For this review, take the finished solid that the model builds, in its own axes (mm). A direction names the side the tool comes from. Coordinates: 2 decimals unless noted, no trailing zeros. Order: outer loops, then holes, each group sorted by start corner. A loop starts at its lowest first (then second) coordinate and runs counter-clockwise, first axis right, second up. Notation, with made-up numbers: M -31,23 L 9,23 A13 cw 9,38 Z; hole C 89,76.25 d4. An arc over 180 degrees is marked long. Use CSV: the item, a comma, the result in double quotes.
Autodesk Inventor part; units mm, degrees
ref_plane "YZ Plane" through (0, 0, 0) normal (1, 0, 0) x (0, 1, 0)
ref_plane "XZ Plane" through (0, 0, 0) normal (0, 1, 0) x (-1, 0, 0)
ref_plane "XY Plane" through (0, 0, 0) normal (0, 0, 1) x (1, 0, 0)
ref_plane "Plano de trabajo1" through (0, 0, 0) normal (0, 0, 1) x (1, 0, 0)
sketch "Boceto1" plane through (0, 0, 0) normal (0, 0, 1) x (1, 0, 0)
  line L0 (0, 0) -> (0, -3) construction
  line L1 (20, -3) -> (0, -3) construction
  line L2 (20, 0) -> (20, -3) construction
  line L3 (20, 0) -> (-49, 0)
  line L4 (-49, 0) -> (-49, 85) construction
  line L5 (-49, 85) -> (20, 85) construction
  line L6 (20, 85) -> (20, 0) construction
  line L7 (0, 0) -> (0, -1)
  line L8 (20, -1) -> (20, 0)
  line L9 (18, -3) -> (2, -3)
  arc A0 (0, -1) -> (2, -3) centre (2, -1) ccw
  arc A1 (18, -3) -> (20, -1) centre (18, -1) ccw
  line L10 (20, 0) -> (35.1716, 0)
  line L11 (40, 0) -> (40, 20) construction
  line L12 (40, 20) -> (20, 20) construction
  line L13 (20, 20) -> (20, 0)
  line L14 (-34, 0) -> (-34, -3) construction
  circle A2 centre (-39, 10.2728) radius 1.55
  line L15 (40, 0) -> (20, 20)
  line L16 (20, 20) -> (-49, 20)
  line L17 (-20, 20) -> (-39, 85)
  line L18 (-49, 0) -> (-49, 85)
  line L19 (-39, 85) -> (-49, 85)
  line L20 (40, 0) -> (20, 0)
  circle A3 centre (-42.7477, 80) radius 1.4 construction
  circle A4 centre (-42.7477, 80) radius 1.55
  point P0 (35.1716, 0)
  dimension "d0" = 2
  dimension "d1" = 20
  dimension "d2" = 20
  dimension "d4" = 85
  dimension "d5" = 15
  dimension "d6" = 3.1
  dimension "d8" = 45
  dimension "d9" = 0
  dimension "d12" = 40
  dimension "d13" = 10
  dimension "d28" = 3.1
extrude "Extrusión1" add sketch "Boceto1" along normal blind 3.1
fillet "Empalme1" radius 2 1 edges at (40, 0, 1.55)
fillet "Empalme2" radius 12 1 edges at (-49, 0, 1.55)
fillet "Empalme3" radius 4 1 edges at (20, 20, 1.55)
fillet "Empalme4" radius 12 1 edges at (-20, 20, 1.55)
fillet "Empalme5" radius 5 2 edges at (-39, 85, 1.55) (-49, 85, 1.55)
sketch "Boceto2" plane through (0, 0, 3.1) normal (0, 0, 1) x (1, 0, 0)
  circle A0 centre (15, 15) radius 1.6 construction
  circle A1 centre (5, 15) radius 1.6 construction
  arc A2 (-44, 85) -> (-49, 80) centre (-44, 80) ccw construction
  arc A3 (-37.9485, 81.4028) -> (-42.7477, 85) centre (-42.7477, 80) ccw construction
  point P0 (0, 0)
hole "Agujero1" at (5, 15, 3.1) at (15, 15, 3.1) direction (0, 0, -1) diameter 3 end through all
equation "\"d14\" = d28"
properties part number "ParedLateralGrua1"
Item 1: Clearance check with flat-ended pins moving along their axes: pin 1 Ø1.6 at (x, z) = (-20, 2) entering from -Y; pin 2 Ø0.5 at (y, z) = (-0.5, 2.5) entering from -X; pin 3 Ø0.8 at (y, z) = (-0.5, 1) entering from +X. State where each tip first meets the part, or that it passes through.
Solutions:
pin 1,"y = 0"
pin 2,"x = 0"
pin 3,"x = 20"
Item 2: For faces 1 (the face through (-18, 0, 2)), 2 (the face through (27, 0, 2)), 3 (the face through (19.89, 19.69, 1.57)), list the 3-axis set-ups (+Z, -Z, +X, -X, +Y, -Y) from which the entire face can be reached by the end or side of a thin tool; tool diameter is ignored.
Solutions:
face 1,"+Z, -Z, -X, -Y"
face 2,"+Z, -Z, +X, -Y"
face 3,"+Z, -Z, +X, +Y"
Item 3: To check wall thickness, follow line 1 along X through (y, z) = (15, 2.2); line 2 along Y through (x, z) = (-9, 0.3); line 3 along Y through (x, z) = (28, 1.9). State the ranges of each line that lie inside material, in increasing order. Write a range as [from, to].
Solutions:
line 1,"[-49, 3.5], [6.5, 13.5], [16.5, 25]"
line 2,"[0, 20]"
line 3,"[0, 12]"
Item 4: Add section D-D on x = 27. State the section outline as (y, z) points, and give its area (3 significant figures).
Solutions:
outline,"M 0,0 L 13,0 L 13,3.1 L 0,3.1 Z"
area,"40.3 mm^2"
Item 5: Add section A-A on y = 15. State the section outline as (x, z) points.
Solutions:
outline,"M -49,0 L 3.5,0 L 3.5,3.1 L -49,3.1 Z; M 6.5,0 L 13.5,0 L 13.5,3.1 L 6.5,3.1 Z; M 16.5,0 L 25,0 L 25,3.1 L 16.5,3.1 Z"
Item 6: Add section C-C on z = 0.6. State the section outline as (x, y) points, and give its area (3 significant figures).
Solutions:
outline,"M -49,12 A12 ccw -37,0 L 0,0 L 0,-1 A2 ccw 2,-3 L 18,-3 A2 ccw 20,-1 L 20,0 L 35.17,0 A2 ccw 36.59,3.41 L 21.17,18.83 A4 ccw 18.34,20 L -11.01,20 A12 cw -22.52,28.63 L -37.95,81.4 A5 ccw -42.75,85 L -44,85 A5 ccw -49,80 Z; hole C -42.75,80 d3.1; hole C -39,10.27 d3.1; hole C 5,15 d3; hole C 15,15 d3"
area,"2,850 mm^2"
Item 7: Draft analysis for pull direction Y (two halves, no side actions). For faces 4 (the face through (10, -3, 2)), 5 (the face through (4.93, 16.5, 1.53)), 6 (the face through (-49, 46, 2)), state which applies: released by +Y, released by -Y, zero draft, split by the parting line, or undercut.
Solutions:
face 4,"released by -Y"
face 5,"undercut"
face 6,"zero draft"
Item 8: Add section B-B on x = 5. State the section outline as (y, z) points.
Solutions:
outline,"M -3,0 L 13.5,0 L 13.5,3.1 L -3,3.1 Z; M 16.5,0 L 20,0 L 20,3.1 L 16.5,3.1 Z"
